```python
from build123d import *

# Parameters (mm, degrees)
ESBO_O1_W                  = 100
ESBO_O1_H                  = 60
RESSALTO_EXTRUS_O1_DEPTH   = 1
ESBO_O2_W                  = 3
ESBO_O2_H                  = 3
RESSALTO_EXTRUS_O2_DEPTH   = 14
CORTE_EXTRUS_O1_DEPTH      = 73.083285164
CORTE_EXTRUS_O1_DEPTH_BACK = 73.083285164
ESBO_O3_R                  = 1.025
FILETE1_R                  = 1
FILETE2_R                  = 1


with BuildPart() as part:
    # Esboço1 → Ressalto-extrusão1 (new body)
    with BuildSketch(Plane.XY):
        Rectangle(ESBO_O1_W, ESBO_O1_H)
    extrude(amount=RESSALTO_EXTRUS_O1_DEPTH)

    # Esboço2 → Ressalto-extrusão2 (add)
    with BuildSketch(Plane.XY):
        with Locations((17.3, 18.5)):
            Rectangle(ESBO_O2_W, ESBO_O2_H)
        with Locations((17.3, -18.5)):
            Rectangle(ESBO_O2_W, ESBO_O2_H)
        with Locations((-17.3, -18.5)):
            Rectangle(ESBO_O2_W, ESBO_O2_H)
        with Locations((-17.3, 18.5)):
            Rectangle(ESBO_O2_W, ESBO_O2_H)
    extrude(amount=RESSALTO_EXTRUS_O2_DEPTH)

    # Esboço3 → Corte-extrusão1 (cut, two sides: drawn at the far end of the back side and taken through both)
    with BuildSketch(Plane(origin=(0, -20, 0), x_dir=(-1, 0, 0), z_dir=(0, -1, 0)).offset(-CORTE_EXTRUS_O1_DEPTH_BACK)):
        with Locations(Location((-17.3, -11.5, 0), (0, 0, 90))):
            Circle(ESBO_O3_R)
        with Locations(Location((17.3, -11.5, 0), (0, 0, 90))):
            Circle(ESBO_O3_R)
    extrude(amount=CORTE_EXTRUS_O1_DEPTH + CORTE_EXTRUS_O1_DEPTH_BACK, mode=Mode.SUBTRACT)

    # Filete1
    filete1_edges = [part.edges().sort_by_distance(p)[0] for p in [
        (15.8, -18.5, 14),
    ]]
    fillet(filete1_edges, radius=FILETE1_R)

    # Filete2
    filete2_edges = [part.edges().sort_by_distance(p)[0] for p in [
        (18.8, 18.5, 14),
        (15.8, 18.5, 14),
        (18.8, -18.5, 14),
    ]]
    fillet(filete2_edges, radius=FILETE2_R)


solid = part.part
```
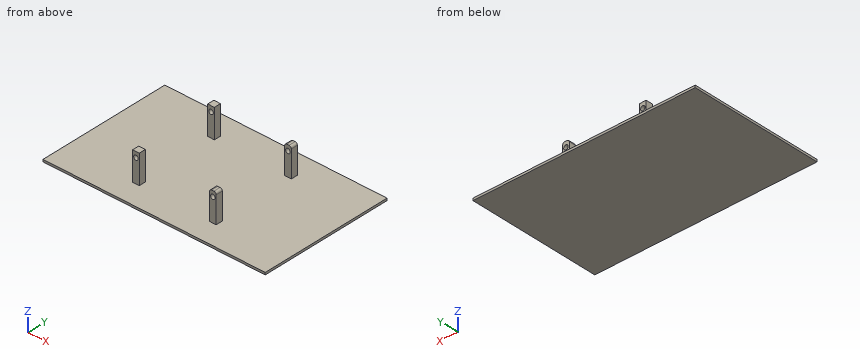
Geometry: final body of the model. Coordinates: model frame, mm. Coordinates: 2 decimals unless noted, no trailing zeros. Order: outer loops, then holes, each group sorted by start corner. A loop starts at its lowest first (then second) coordinate and runs counter-clockwise, first axis right, second up. Notation, with made-up numbers: M 66,20.5 L 72,20.5 A26 ccw 72,59.5 Z; hole C -11,11.5 d7. An arc over 180 degrees is marked long. Answer in a Markdown table with one row per item. Add a question column.
Q1. Section query B-B on z = 3. Return the cut outline in (x, y).
Q2. Section query A-A on x = -17.3. Return the cut outline in (y, z) (3 decimals), and give its area (3 significant figures).
Q3. Line query: L1, parallel to X at y = 18.35, z = 11.5 (3 decimals); L2, parallel to Z at x = -10, y = 27.5; L3, parallel to X at y = -18, z = 5. Output: solid intervals per line, ascending.
Q4. Contact query for flat-ended pins moving along their axis: P1, Ø1.5, axis at x = -17, z = 8, coming from the -Y side; P2, Ø0.9, axis at y = 19, z = 8.5, coming from the +X side; P3, Ø2.5, axis at y = 19, z = 6, coming from the -X side. Output: stop coordinate, or through.
Q5. Section query C-C on y = 18. Return the cut outline in (x, z) (3 decimals), and give its area (3 significant figures).
Q6. Section query D-D on z = 11.5. Count the separate pieces of the cut face and the enclosed holes in it, and give its area (3 significant figures).
Completed:
| question | item | result |
|---|---|---|
| 1 | outline | M -18.8,-20 L -15.8,-20 L -15.8,-17 L -18.8,-17 Z; M -18.8,17 L -15.8,17 L -15.8,20 L -18.8,20 Z; M 15.8,-20 L 18.8,-20 L 18.8,-17 L 15.8,-17 Z; M 15.8,17 L 18.8,17 L 18.8,20 L 15.8,20 Z |
| 2 | outline | M -30,0 L 30,0 L 30,1 L 20,1 L 20,10.475 L 17,10.475 L 17,1 L -17,1 L -17,10.475 L -20,10.475 L -20,1 L -30,1 Z; M -20,12.525 L -17,12.525 L -17,14 L -20,14 Z; M 17,12.525 L 20,12.525 L 20,14 L 17,14 Z |
| 2 | area | 126 mm2 |
| 3 | L1 | x = -18.8 to -18.325, -16.275 to -15.8, 15.8 to 16.275, 18.325 to 18.8 |
| 3 | L2 | z = 0 to 1 |
| 3 | L3 | x = -18.8 to -15.8, 15.8 to 18.8 |
| 4 | P1 | stops at y = -20 |
| 4 | P2 | stops at x = 18.8 |
| 4 | P3 | stops at x = -18.8 |
| 5 | outline | M -50,0 L 50,0 L 50,1 L 18.8,1 L 18.8,13 A1 ccw 17.8,14 L 16.8,14 A1 ccw 15.8,13 L 15.8,1 L -15.8,1 L -15.8,14 L -18.8,14 L -18.8,1 L -50,1 Z; hole C -17.3,11.5 d2.05; hole C 17.3,11.5 d2.05 |
| 5 | area | 171 mm2 |
| 6 | separate pieces | 8 |
| 6 | enclosed holes | 0 |
| 6 | area | 11.4 mm2 |
